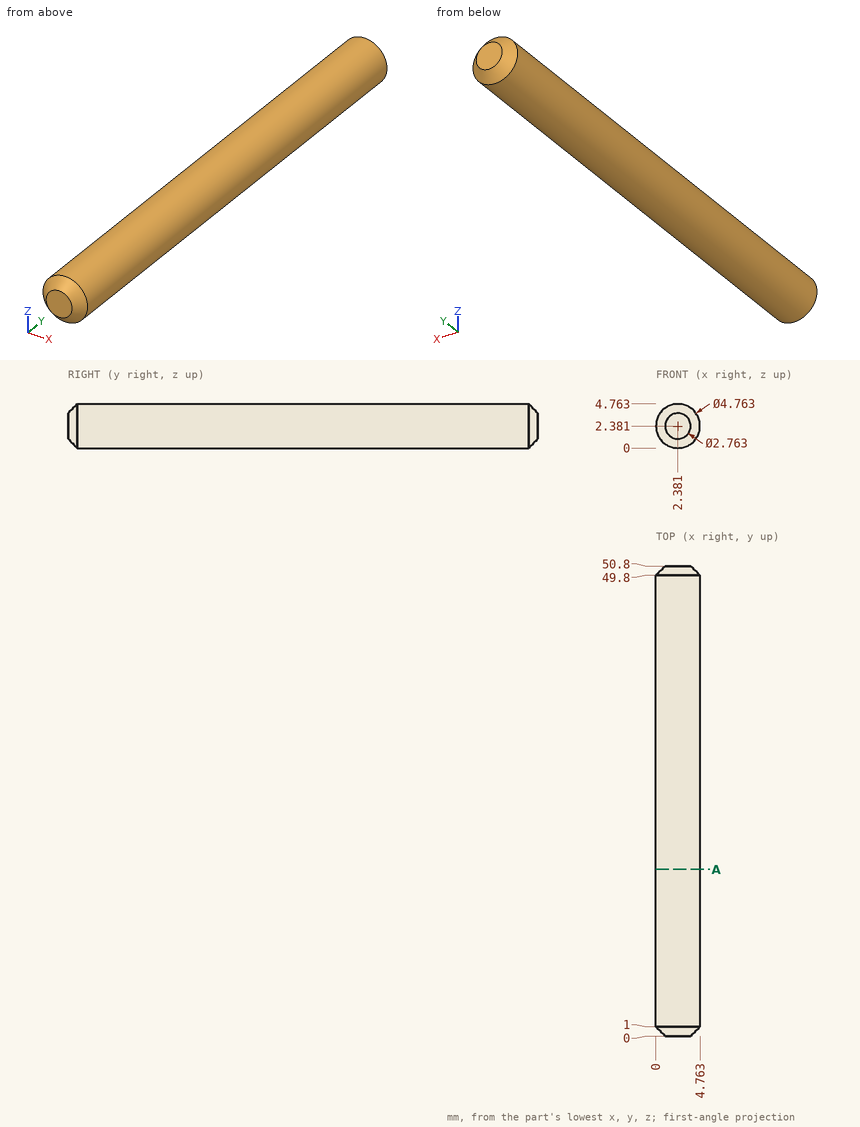
Input: dimensioned drawing with shaded views. Units: mm. Origin: part minimum x, y, z. Give positions to 0.01 mm unless a question says otherwise; leave off trailing zeros. Write each loop counter-clockwise with the first axis right and the second up, starting at its lowest first coordinate (ties: lowest second). Pieces come first, ordered by that corner, then holes.
1. Line query: probe 1 along Z at (x, y) = (2.5, 35.5); probe 2 along X at (y, z) = (19, 2.7); probe 3 along Y at (x, z) = (1.25, 4.1) (1 decimal). Output: solid intervals per line, ascending.
2. Pin query (flat end, axial travel): P1, Ø2, axis at x = 4, y = 30.5, coming from the -Z side. Return the tip coordinate at first contact, or that it passes through.
3. Section query A-A, the plane y = 18. Return loops of the section in (x, z), then the cut area to 3 significant figures.
Computed:
1. probe 1: z = 0 to 4.76
1. probe 2: x = 0.02 to 4.74
1. probe 3: y = 0.7 to 50.1
2. P1: stops at z = 0.08
3. outline: circle Ø4.76 at (2.38, 2.38)
3. area: 17.8 mm2
